from build123d import *

# Parameters (mm, degrees)
CROQUIS3_W              = 30
CROQUIS3_H              = 23
CROQUIS3_R              = 2.55
SALIENTE_EXTRUIR2_DEPTH = 2
CROQUIS5_W              = 8
CROQUIS5_H              = 8
CROQUIS5_R              = 2.55
SALIENTE_EXTRUIR3_DEPTH = 12
SALIENTE_EXTRUIR4_DEPTH = 23
CROQUIS7_R              = 3.75
CORTAR_EXTRUIR1_DEPTH   = 15
CORTAR_EXTRUIR7_START   = -3
CORTAR_EXTRUIR7_DEPTH   = 20
CORTAR_EXTRUIR8_START   = 2
CROQUIS14_W             = 8.13201816
CROQUIS14_H             = 9.468544415
CORTAR_EXTRUIR8_DEPTH   = 25
CROQUIS15_W             = 24.194573687
CROQUIS15_H             = 9.468544415
CORTAR_EXTRUIR9_DEPTH   = 1.933991
REDONDEO1_R             = 3


with BuildPart() as part:
    # Croquis3 → Saliente-Extruir2 (new body)
    with BuildSketch(Plane.XY):
        with Locations((-48.169014085, 19.436619718)):
            Rectangle(CROQUIS3_W, CROQUIS3_H)
        with Locations((-59.169014085, 26.936619718)):
            Circle(CROQUIS3_R, mode=Mode.SUBTRACT)
        with Locations(Location((-59.169014085, 11.936619718, 0), (0, 0, 180))):
            Circle(CROQUIS3_R, mode=Mode.SUBTRACT)
    extrude(amount=SALIENTE_EXTRUIR2_DEPTH)

    # Croquis5 → Saliente-Extruir3 (add)
    # profile 1 of 2: a face of its own
    with BuildSketch(Plane.XY.offset(2)):
        with Locations((-59.169014085, 11.936619718)):
            Rectangle(CROQUIS5_W, CROQUIS5_H)
        with Locations(Location((-59.169014085, 11.936619718, 0), (0, 0, 180))):
            Circle(CROQUIS5_R, mode=Mode.SUBTRACT)
    # profile 2 of 2: a face of its own
    with BuildSketch(Plane.XY.offset(2)):
        with Locations((-59.169014085, 26.936619718)):
            Rectangle(CROQUIS5_W, CROQUIS5_H)
        with Locations(Location((-59.169014085, 26.936619718, 0), (0, 0, 180))):
            Circle(CROQUIS5_R, mode=Mode.SUBTRACT)
    extrude(amount=SALIENTE_EXTRUIR3_DEPTH)

    # Croquis6 → Saliente-Extruir4 (add)
    with BuildSketch(Plane(origin=(0, 30.936619718, 0), x_dir=(1, 0, 0), z_dir=(0, 1, 0))):
        Polygon((-63.169014085, -14), (-68.299316234, -28.095389312), (-79.575627684, -23.991147592), (-63.169014085, 0), align=None)
    extrude(amount=-SALIENTE_EXTRUIR4_DEPTH)

    # Croquis7 → Cortar-Extruir1 (cut)
    with BuildSketch(Plane(origin=(-17.019186352, 0, 46.759830198), x_dir=(0.9396926207859082, 0, 0.3420201433256694), z_dir=(-0.3420201433256694, 0, 0.9396926207859083))):
        with Locations((-60.571174391, 19.436619718)):
            Circle(CROQUIS7_R)
    extrude(amount=-CORTAR_EXTRUIR1_DEPTH, mode=Mode.SUBTRACT)

    # Croquis13 → Cortar-Extruir7 (cut)
    with BuildSketch(Plane(origin=(-17.019186352, 0, 46.759830198), x_dir=(0.9396926207859082, 0, 0.3420201433256694), z_dir=(-0.3420201433256694, 0, 0.9396926207859083)).offset(CORTAR_EXTRUIR7_START)):
        Polygon((-60.571174391, 14.702347511), (-56.471174391, 17.069483615), (-56.471174391, 21.803755822), (-60.571174391, 24.170891926), (-64.671174391, 21.803755822), (-64.671174391, 17.069483615), align=None)
    extrude(amount=-CORTAR_EXTRUIR7_DEPTH, mode=Mode.SUBTRACT)

    # Croquis14 → Cortar-Extruir8 (cut)
    with BuildSketch(Plane(origin=(-15.993125922, 0, 43.940752336), x_dir=(-0.9396926207859081, 0, -0.34202014332566977), z_dir=(0.3420201433256697, 0, -0.939692620785908)).offset(CORTAR_EXTRUIR8_START)):
        with Locations((60.571174391, 19.436619719)):
            Rectangle(CROQUIS14_W, CROQUIS14_H)
    extrude(amount=CORTAR_EXTRUIR8_DEPTH, mode=Mode.SUBTRACT)

    # Croquis15 → Cortar-Extruir9 (cut)
    with BuildSketch(Plane(origin=(-53.097486879, 0, -19.325904738), x_dir=(-0.34202014332566977, 0, 0.9396926207859081), z_dir=(-0.939692620785908, 0, -0.3420201433256697))):
        with Locations((32.663485099, 19.436619719)):
            Rectangle(CROQUIS15_W, CROQUIS15_H)
    extrude(amount=-CORTAR_EXTRUIR9_DEPTH, mode=Mode.SUBTRACT)

    # Redondeo1
    # the kernel refuses this fillet: 3 mm, written as the material it takes off along each edge
    with BuildSketch(Plane(origin=(-70.092333667, 10.936619718, 24.250251019), x_dir=(0.9396926207859081, 0, 0.34202014332566966), z_dir=(0, -1, 0))) as redondeo1_piece_1_section:
        Polygon((0, 0), (REDONDEO1_R * 1.02, 0), (REDONDEO1_R * 1.02, REDONDEO1_R * 1.02), (0, REDONDEO1_R * 1.02), align=None)
    redondeo1_piece_1 = extrude(amount=REDONDEO1_R * 1.02, mode=Mode.PRIVATE)
    redondeo1_piece_1 = redondeo1_piece_1 - Plane(origin=(-70.092333667, 10.936619718, 24.250251019), x_dir=(-0.4226182617406987, 0, -0.9063077870366504), z_dir=(0, -1, 0)) * Sphere(REDONDEO1_R, mode=Mode.PRIVATE)
    add(redondeo1_piece_1, mode=Mode.SUBTRACT)
    with BuildSketch(Plane(origin=(-74.917413437, 10.936619718, 22.494065605), x_dir=(-0.3420201433256695, 0, 0.9396926207859081), z_dir=(0, -1, 0))) as redondeo1_piece_2_section:
        Polygon((0, 0), (REDONDEO1_R * 1.02, 0), (REDONDEO1_R * 1.02, REDONDEO1_R * 1.31418750187), (-REDONDEO1_R * 0.253089576506, REDONDEO1_R * 0.988102052555), align=None)
    redondeo1_piece_2 = extrude(amount=REDONDEO1_R * 1.02, mode=Mode.PRIVATE)
    redondeo1_piece_2 = redondeo1_piece_2 - Plane(origin=(-74.917413437, 10.936619718, 22.494065605), x_dir=(0.9520405381935744, 0, -0.30597191641732324), z_dir=(0, -1, 0)) * Sphere(REDONDEO1_R, mode=Mode.PRIVATE)
    add(redondeo1_piece_2, mode=Mode.SUBTRACT)
    with BuildSketch(Plane(origin=(-70.092333667, 27.936619718, 24.250251019), x_dir=(0.9396926207859081, 0, 0.34202014332566966), z_dir=(0, 1, 0))) as redondeo1_piece_3_section:
        Polygon((0, 0), (REDONDEO1_R * 1.02, 0), (REDONDEO1_R * 1.02, -REDONDEO1_R * 1.02), (0, -REDONDEO1_R * 1.02), align=None)
    redondeo1_piece_3 = extrude(amount=REDONDEO1_R * 1.02, mode=Mode.PRIVATE)
    redondeo1_piece_3 = redondeo1_piece_3 - Plane(origin=(-70.092333667, 27.936619718, 24.250251019), x_dir=(-0.4226182617406987, 0, -0.9063077870366504), z_dir=(0, 1, 0)) * Sphere(REDONDEO1_R, mode=Mode.PRIVATE)
    add(redondeo1_piece_3, mode=Mode.SUBTRACT)
    with BuildSketch(Plane(origin=(-74.917413437, 27.936619718, 22.494065605), x_dir=(-0.3420201433256695, 0, 0.9396926207859081), z_dir=(0, 1, 0))) as redondeo1_piece_4_section:
        Polygon((0, 0), (REDONDEO1_R * 1.02, 0), (REDONDEO1_R * 1.02, -REDONDEO1_R * 1.31418750187), (-REDONDEO1_R * 0.253089576506, -REDONDEO1_R * 0.988102052555), align=None)
    redondeo1_piece_4 = extrude(amount=REDONDEO1_R * 1.02, mode=Mode.PRIVATE)
    redondeo1_piece_4 = redondeo1_piece_4 - Plane(origin=(-74.917413437, 27.936619718, 22.494065605), x_dir=(0.9520405381935744, 0, -0.30597191641732324), z_dir=(0, 1, 0)) * Sphere(REDONDEO1_R, mode=Mode.PRIVATE)
    add(redondeo1_piece_4, mode=Mode.SUBTRACT)
    with BuildSketch(Plane(origin=(-55.169014085, 7.936619718, 2), x_dir=(0, 1, 0), z_dir=(0, 0, 1)), Plane(origin=(-55.169014085, 15.936619718, 2), x_dir=(-1, 0, 0), z_dir=(0, 0, 1)), Plane(origin=(-55.169014085, 30.936619718, 2), x_dir=(-1, 0, 0), z_dir=(0, 0, 1))) as redondeo1_piece_5:
        with BuildLine():
            CenterArc((REDONDEO1_R, REDONDEO1_R), REDONDEO1_R, 180, 90)
            Line((0, REDONDEO1_R), (0, 0))
            Line((0, 0), (REDONDEO1_R, 0))
        make_face()
    extrude(amount=19.5, mode=Mode.SUBTRACT)
    with BuildSketch(Plane(origin=(-55.169014085, 22.936619718, 2), x_dir=(-1, 0, 0), z_dir=(0, 0, 1))) as redondeo1_piece_6:
        with BuildLine():
            CenterArc((REDONDEO1_R, -REDONDEO1_R), REDONDEO1_R, 90, 90)
            Line((0, -REDONDEO1_R), (0, 0))
            Line((0, 0), (REDONDEO1_R, 0))
        make_face()
    extrude(amount=19.5, mode=Mode.SUBTRACT)
    with BuildSketch(Plane(origin=(-60.60386301, 7.936619718, 6.952305344), x_dir=(0, 1, 0), z_dir=(-0.34202014332566966, 0, 0.9396926207859081))) as redondeo1_piece_7_section:
        with BuildLine():
            CenterArc((REDONDEO1_R, REDONDEO1_R), REDONDEO1_R, 180, 90)
            Line((0, REDONDEO1_R), (0, 0))
            Line((0, 0), (REDONDEO1_R, 0))
        make_face()
    redondeo1_piece_7 = extrude(amount=19.5, mode=Mode.PRIVATE)
    redondeo1_piece_7 = split(redondeo1_piece_7, bisect_by=Plane(origin=(-65.882719938, 8.612486754, 14), z_dir=(0, 0, 1)), keep=Keep.TOP, mode=Mode.PRIVATE)
    add(redondeo1_piece_7, mode=Mode.SUBTRACT)
    with BuildSketch(Plane(origin=(-71.118394097, 7.936619718, 27.069328882), x_dir=(0.3420201433256695, 0, -0.9396926207859081), z_dir=(-0.9396926207859081, 0, -0.3420201433256695))) as redondeo1_piece_8:
        with BuildLine():
            CenterArc((REDONDEO1_R, -REDONDEO1_R), REDONDEO1_R, 90, 90)
            Line((0, -REDONDEO1_R), (0, 0))
            Line((0, 0), (REDONDEO1_R, 0))
        make_face()
    extrude(amount=5.134742642, mode=Mode.SUBTRACT)
    with BuildSketch(Plane(origin=(-68.299316234, 27.936619718, 28.095389312), x_dir=(0.34202014332566905, 0, -0.9396926207859082), z_dir=(0, -1, 0)), Plane(origin=(-33.169014085, 7.936619718, -7.5), x_dir=(-1, 0, 0), z_dir=(0, 0, 1))) as redondeo1_piece_9:
        with BuildLine():
            CenterArc((REDONDEO1_R, -REDONDEO1_R), REDONDEO1_R, 90, 90)
            Line((0, -REDONDEO1_R), (0, 0))
            Line((0, 0), (REDONDEO1_R, 0))
        make_face()
    extrude(amount=17, mode=Mode.SUBTRACT)
    with BuildSketch(Plane(origin=(-77.393738361, 7.936619718, 20.800603214), x_dir=(0.8254416413123481, 0, 0.5644874638001954), z_dir=(0.5644874638001954, 0, -0.8254416413123482))) as redondeo1_piece_10:
        with BuildLine():
            CenterArc((REDONDEO1_R, -REDONDEO1_R), REDONDEO1_R, 90, 90)
            Line((0, -REDONDEO1_R), (0, 0))
            Line((0, 0), (REDONDEO1_R, 0))
        make_face()
    extrude(amount=32.699362587, mode=Mode.SUBTRACT)
    with BuildSketch(Plane(origin=(-79.575627684, 27.936619718, 23.991147592), x_dir=(0.9396926207859081, 0, 0.3420201433256696), z_dir=(0, -1, 0))) as redondeo1_piece_11:
        with BuildLine():
            CenterArc((REDONDEO1_R * 1.28841911948, -REDONDEO1_R), REDONDEO1_R, 90, 104.366707449)
            Line((REDONDEO1_R * 0.319691616972, -REDONDEO1_R * 1.24812703579), (0, 0))
            Line((0, 0), (REDONDEO1_R * 1.28841911948, 0))
        make_face()
    extrude(amount=17, mode=Mode.SUBTRACT)
    with BuildSketch(Plane(origin=(-77.393738361, 30.936619718, 20.800603214), x_dir=(0.8254416413123481, 0, 0.5644874638001954), z_dir=(0.5644874638001954, 0, -0.8254416413123482))) as redondeo1_piece_12:
        with BuildLine():
            CenterArc((REDONDEO1_R, REDONDEO1_R), REDONDEO1_R, 180, 90)
            Line((0, REDONDEO1_R), (0, 0))
            Line((0, 0), (REDONDEO1_R, 0))
        make_face()
    extrude(amount=32.699362587, mode=Mode.SUBTRACT)
    with BuildSketch(Plane(origin=(-71.118394097, 30.936619718, 27.069328882), x_dir=(0.3420201433256695, 0, -0.9396926207859081), z_dir=(-0.9396926207859081, 0, -0.3420201433256695))) as redondeo1_piece_13:
        with BuildLine():
            CenterArc((REDONDEO1_R, REDONDEO1_R), REDONDEO1_R, 180, 90)
            Line((0, REDONDEO1_R), (0, 0))
            Line((0, 0), (REDONDEO1_R, 0))
        make_face()
    extrude(amount=5.134742642, mode=Mode.SUBTRACT)
    with BuildSketch(Plane(origin=(-60.60386301, 30.936619718, 6.952305344), x_dir=(-0.9396926207859081, 0, -0.3420201433256697), z_dir=(-0.34202014332566966, 0, 0.9396926207859081))) as redondeo1_piece_14_section:
        with BuildLine():
            CenterArc((REDONDEO1_R, REDONDEO1_R), REDONDEO1_R, 180, 90)
            Line((0, REDONDEO1_R), (0, 0))
            Line((0, 0), (REDONDEO1_R, 0))
        make_face()
    redondeo1_piece_14 = extrude(amount=19.5, mode=Mode.PRIVATE)
    redondeo1_piece_14 = split(redondeo1_piece_14, bisect_by=Plane(origin=(-65.882719938, 30.260752682, 14), z_dir=(0, 0, 1)), keep=Keep.TOP, mode=Mode.PRIVATE)
    add(redondeo1_piece_14, mode=Mode.SUBTRACT)
    with BuildSketch(Plane(origin=(-33.169014085, 30.936619718, -7.5), x_dir=(-1, 0, 0), z_dir=(0, 0, 1))) as redondeo1_piece_15:
        with BuildLine():
            CenterArc((REDONDEO1_R, REDONDEO1_R), REDONDEO1_R, 180, 90)
            Line((0, REDONDEO1_R), (0, 0))
            Line((0, 0), (REDONDEO1_R, 0))
        make_face()
    extrude(amount=17, mode=Mode.SUBTRACT)


solid = part.part
Input: part model. Units: mm. Frame: model coordinates. A direction names the side the tool comes from. Round coordinates to 2 decimals unless told otherwise and drop trailing zeros. Order: outer loops, then holes, each group sorted by start corner. A loop starts at its lowest first (then second) coordinate and runs counter-clockwise, first axis right, second up. Notation, with made-up numbers: (-20, 52.25) - (16, 52.25) arc R16 cw to (16, 71.25) - close; hole circle Ø9 at (-21, 35). An arc over 180 degrees is marked (long way). Answer as a JSON object with one key per item and string values. Group by question number.
(1) Material intervals for probe 1 along Y at (x, z) = (-61.5, 4); probe 2 along Y at (x, z) = (-69, 13.5); probe 3 along Z at (x, y) = (-48.5, 28.75), sorted ascending. Write a range as from..to.
(2) Draft query along X for faces 1 (the face through (-56.071, 23.792, 7.916)), 2 (the face through (-69.065, 8.792, 10.22)), 3 (the face through (-74.389, 23.004, 21.375)). Return one class per face: released by +X, released by -X, zero draft, split by the parting line, or undercut.
(3) Cut plane C-C (x = -39). Return loops of the section in (y, z).
(4) Pin query (flat end, axial travel): P1, Ø1, axis at y = 12.5, z = 7.5, coming from the +X side; P2, Ø2, axis at x = -41.5, y = 21.5, coming from the -Z side; P3, Ø3, axis at y = 26, z = 4, coming from the -X side; P4, Ø7, axis at x = -41, y = 19.5, coming from the +Z side. Return the tip coordinate at first contact, or that it passes through.
(5) Cut plane A-A (y = 29). Return loops of the section in (x, z), then the cut area to 3 significant figures.
(6) Reachability of faces 4 (the face through (-56.02, 30.03, 7.92)), 5 (the face through (-76.02, 19.47, 19.78)), 6 (the face through (-68.72, 19.4, 23.7)), 7 (the face through (-59.236, 19.37, 0.326)), 8 (the face through (-74.6, 15.9, 21.8)) from +Z, -Z, +X, -X, +Y, -Y: full face, straight path, thin tool, end or side. Return the list, or none.
(7) Cut plane B-B (z = 6). Count the separate pieces of the cut face and the enclosed holes in it, then the cut area to 3 significant figures.
Here are the results:
{
 "1": {"probe 1": "y = 7.94..10.9, 12.97..14.7, 24.17..25.9, 27.97..30.94", "probe 2": "y = 7.94..14.7, 24.17..30.93", "probe 3": "z = 0..2"},
 "2": {"face 1": "released by +X", "face 2": "released by -X", "face 3": "undercut"},
 "3": {"outline": "(7.94, 0) - (30.94, 0) - (30.94, 2) - (7.94, 2) - close"},
 "4": {"P1": "stops at x = -55.17", "P2": "stops at z = 0", "P3": "stops at x = -66.93", "P4": "stops at z = 2"},
 "5": {"outline": "(-77.23, 20.91) - (-62.93, 0) - (-60.67, 0) - (-60.67, 14) - (-63.38, 14) - (-67.46, 25.21) arc R2.81 ccw to (-71.05, 26.89) - (-75.88, 25.13) arc R2.81 ccw to start; (-57.67, 0) - (-33.36, 0) - (-33.36, 2) - (-55.36, 2) - (-55.36, 14) - (-57.67, 14) - close", "area": "301 mm^2"},
 "6": {"face 4": "+Z, +X, +Y", "face 5": "+X", "face 6": "-Z", "face 7": "-X", "face 8": "none"},
 "7": {"separate pieces": "2", "enclosed holes": "2", "area": "123 mm^2"}
}
